Design review of the part built by this model. Coordinates are the model's own, in mm. Face numbers are marked on the shaded views. A direction names the side the tool comes from. Coordinates: 2 decimals unless noted, no trailing zeros. Loops run counter-clockwise (first coordinate to the right, second up) from the corner with the lowest first, then second, coordinate; pieces in that order, holes last. Notation, with made-up numbers: (-15.75, 32) -> (42.25, 32) arc R6 ccw to (42.25, 37) -> close; hole circle Ø9 at (-24, 83). An arc over 180 degrees is marked (long way). Answer as a JSON object with one key per item and string values.
```python
from build123d import *

# Parameters (mm, degrees)
BOSS_EXTRUDE2_DEPTH = 3
SKETCH5_R           = 3
BOSS_EXTRUDE3_DEPTH = 50


with BuildPart() as part:
    # Sketch4 → Boss-Extrude2 (new, symmetric)
    with BuildSketch(Plane.XY):
        Polygon((0, 6.92820323), (-6, 3.464101615), (-6, -3.464101615), (0, -6.92820323), (6, -3.464101615), (6, 3.464101615), align=None)
    extrude(amount=BOSS_EXTRUDE2_DEPTH, both=True)

    # Sketch5 → Boss-Extrude3 (add)
    with BuildSketch(Plane(origin=(0, 0, -3), x_dir=(-1, 0, 0), z_dir=(0, 0, -1))):
        Circle(SKETCH5_R)
    extrude(amount=BOSS_EXTRUDE3_DEPTH)


solid = part.part
```
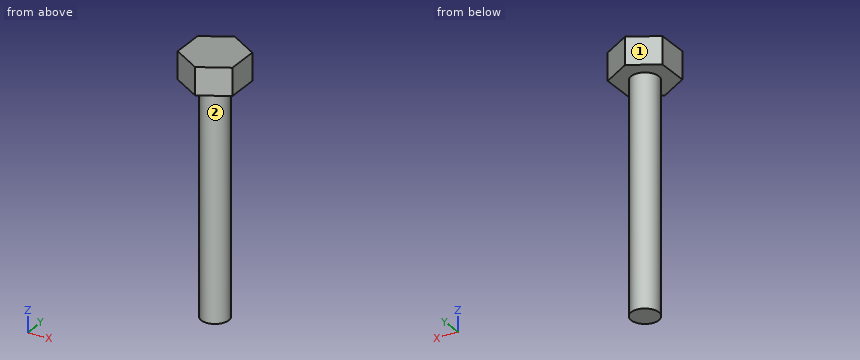
1) Add section A-A, the plane y = 0. Give the boundary of the cut face in (x, z).
Completed:
{"outline": "(-6, -3) -> (-3, -3) -> (-3, -53) -> (3, -53) -> (3, -3) -> (6, -3) -> (6, 3) -> (-6, 3) -> close"}
2) Add section B-B, the plane x = -2.5. Give the boundary of the cut face in (y, z).
Completed:
{"outline": "(-5.48, -3) -> (-1.66, -3) -> (-1.66, -53) -> (1.66, -53) -> (1.66, -3) -> (5.48, -3) -> (5.48, 3) -> (-5.48, 3) -> close"}
3) Wall thickness on probe 1 along X at (y, z) = (0.25, -21.5); probe 2 along Z at (x, y) = (2.5, 2): over which ranges is each line inside the solid? List them lowest first.
Completed:
{"probe 1": "-2.99 to 2.99", "probe 2": "-3 to 3"}
4) Clearance check with flat-ended pins moving along their axes: pin 1 Ø1.5 at (y, z) = (-3, -42.5) entering from +X; pin 2 Ø5 at (x, z) = (-1.5, -3.5) entering from +Y; pin 3 Ø3 at (x, z) = (1.5, -24) entering from -Y. State where each tip first meets the part, or that it passes through.
Completed:
{"pin 1": "x = 1.98", "pin 2": "y = 6.93", "pin 3": "y = -3"}
5) Add section D-D, the plane y = 5.75. Give the boundary of the cut face in (x, z).
Completed:
{"outline": "(-2.04, -3) -> (2.04, -3) -> (2.04, 3) -> (-2.04, 3) -> close"}
6) For the marked faces 1 and 2, list the 3-axis set-ups (+Z, -Z, +X, -X, +Y, -Y) from which the entire face can be reached by the end or side of a thin tool; tool diameter is ignored.
Completed:
{"face 1": "+Z, -Z, -X, +Y", "face 2": "-Z"}
7) Add section C-C, the plane z = -6.5. Give the boundary of the cut face in (x, y), and give its area (3 significant figures).
Completed:
{"outline": "circle Ø6 at (0, 0)", "area": "28.3 mm²"}
